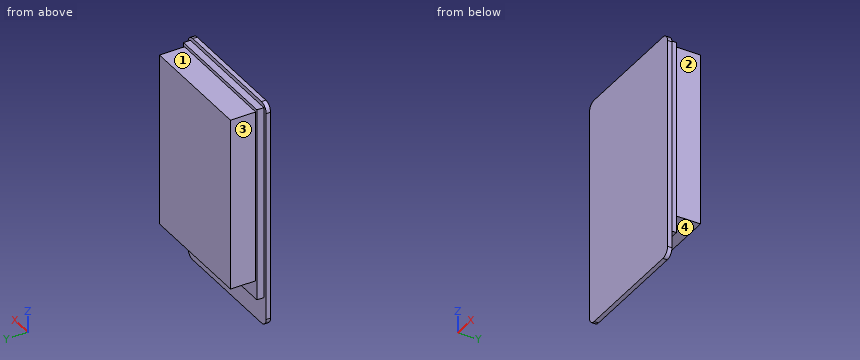
```python
from build123d import *

# Parameters (mm, degrees)
SKETCH_1_W      = 66
SKETCH_1_H      = 114.5
EXTRUDE_1_DEPTH = 2.2
FILLET_1_R      = 4
SKETCH_2_W      = 62
SKETCH_2_H      = 98.3
EXTRUDE_2_DEPTH = 3.5
SKETCH_3_W      = 60
SKETCH_3_H      = 87.364717042
EXTRUDE_3_DEPTH = 12.7


with BuildPart() as part:
    # 스케치1 → 보스-돌출1 (new body)
    with BuildSketch(Plane(origin=(0, 0, 0), x_dir=(1, 0, 0), z_dir=(0, 1, 0))):
        Rectangle(SKETCH_1_W, SKETCH_1_H)
    extrude(amount=EXTRUDE_1_DEPTH)

    # 필렛1
    fillet_1_edges = [part.edges().sort_by_distance(p)[0] for p in [
        (-33, 1.1, -57.25),
        (33, 1.1, -57.25),
        (33, 1.1, 57.25),
        (-33, 1.1, 57.25),
    ]]
    fillet(fillet_1_edges, radius=FILLET_1_R)

    # 스케치2 → 보스-돌출2 (add)
    with BuildSketch(Plane(origin=(0, 2.2, 0), x_dir=(1, 0, 0), z_dir=(0, 1, 0))):
        with Locations((0, -6.1)):
            Rectangle(SKETCH_2_W, SKETCH_2_H)
    extrude(amount=EXTRUDE_2_DEPTH)

    # 스케치3 → 보스-돌출3 (add)
    with BuildSketch(Plane(origin=(0, 5.7, 0), x_dir=(1, 0, 0), z_dir=(0, 1, 0))):
        with Locations((0, -9.917641479)):
            Rectangle(SKETCH_3_W, SKETCH_3_H)
    extrude(amount=EXTRUDE_3_DEPTH)


solid = part.part
```
Design review of the part built by this model. Coordinates are the model's own, in mm. Face numbers are marked on the shaded views. A direction names the side the tool comes from. Give positions to 0.01 mm unless a question says otherwise; leave off trailing zeros. Loops run counter-clockwise (first coordinate to the right, second up) from the corner with the lowest first, then second, coordinate; pieces in that order, holes last. Notation, with made-up numbers: M 37.25,54 L 50.25,54 A28 cw 50.25,72 Z; hole C 50,50.25 d9. An arc over 180 degrees is marked long. Return JSON: item names as keys, results as strings. Group by question number.
Item 1: We need section B-B (z = 22). Give the boundary of the cut face in (x, y).
Item 2: We need section C-C (y = 7). Give the boundary of the cut face in (x, z), and give its area (3 significant figures).
Item 3: Tool access review of the marked faces 1, 2, 3 and 4: name each direction out of +Z, -Z, +X, -X, +Y, -Y from which nothing blocks a thin tool from reaching the whole face with its end or side.
Item 4: We need section D-D (z = -45.5). Give the boundary of the cut face in (x, y).
Item 5: For probe 1 along X at (y, z) = (11, 28.5); probe 2 along Z at (x, y) = (-23.5, 5.75); probe 3 along Z at (x, y) = (-10, 5.25), list the stretches that pass through material, from the lowest coordinate up.
Item 6: We need section A-A (x = 0). Give the boundary of the cut face in (y, z), and give its area (3 significant figures).
Item 7: Insertion check: pin 1 Ø1 at (x, y) = (-10.5, 4) entering from -Z; pin 2 Ø10 at (x, y) = (-23, 8) entering from +Z; pin 3 Ø10 at (y, z) = (12, 30.5) entering from +X. Each pin has a flat end and moves straight along its axis. Give the tip position at first contact, or say it passes through.
Output:
{
 "1": {"outline": "M -33,0 L 33,0 L 33,2.2 L 31,2.2 L 31,5.7 L 30,5.7 L 30,18.4 L -30,18.4 L -30,5.7 L -31,5.7 L -31,2.2 L -33,2.2 Z"},
 "2": {"outline": "M -30,-33.76 L 30,-33.76 L 30,53.6 L -30,53.6 Z", "area": "5,240 mm^2"},
 "3": {"face 1": "+Z, +X, -X, +Y", "face 2": "+Z, -Z, +X, +Y", "face 3": "+Z, -Z, -X, +Y", "face 4": "-Z, +X, -X, +Y"},
 "4": {"outline": "M -33,0 L 33,0 L 33,2.2 L -33,2.2 Z"},
 "5": {"probe 1": "x = -30 to 30", "probe 2": "z = -33.76 to 53.6", "probe 3": "z = -43.05 to 55.25"},
 "6": {"outline": "M 0,-57.25 L 2.2,-57.25 L 2.2,-43.05 L 5.7,-43.05 L 5.7,-33.76 L 18.4,-33.76 L 18.4,53.6 L 5.7,53.6 L 5.7,55.25 L 2.2,55.25 L 2.2,57.25 L 0,57.25 Z", "area": "1,710 mm^2"},
 "7": {"pin 1": "stops at z = -43.05", "pin 2": "stops at z = 55.25", "pin 3": "stops at x = 30"}
}
